from build123d import *

# Parameters (mm, degrees)
F0_R     = 40
F1_DEPTH = 10
F2_SIZE  = 2
F3_R     = 22.145473903
F4_DEPTH = 25
F6_D     = 10
F7_R     = 2
F8_SIZE  = 5


with BuildPart() as f1:
    # F0 (on Top) → F1 (new body)
    with BuildSketch(Plane.XY):
        with Locations((-1.4435499907, 0.3608763218)):
            Circle(F0_R)
    extrude(amount=F1_DEPTH)

    # F2
    f2_edges = [f1.edges().sort_by_distance(p)[0] for p in [
        (-41.44355, 0.360876, 10),
    ]]
    chamfer(f2_edges, length=F2_SIZE)

    # F3 (on face) → F4 (join)
    with BuildSketch(Plane.XY.offset(10)):
        Circle(F3_R)
    extrude(amount=F4_DEPTH)

    # F6 (through all)
    with Locations(Plane.XY.offset(35)):
        with Locations((0, 0)):
            Hole(F6_D / 2)

    # F7
    f7_edges = [f1.edges().sort_by_distance(p)[0] for p in [
        (-41.44355, 0.360876, 0),
        (-22.145474, 0, 35),
        (-5, 0, 0),
    ]]
    fillet(f7_edges, radius=F7_R)

    # F8
    f8_edges = [f1.edges().sort_by_distance(p)[0] for p in [
        (22.145474, 0, 21.5),
        (-22.145474, 0, 33),
        (-22.145474, 0, 10),
    ]]
    chamfer(f8_edges, length=F8_SIZE)


solid = f1.part
Read the model definition and answer for the solid it produces. Units are mm, in the model's axes. A direction names the side the tool comes from. Coordinates: 2 decimals unless noted, no trailing zeros. Write each loop counter-clockwise with the first axis right and the second up, starting at its lowest first coordinate (ties: lowest second). Pieces come first, ordered by that corner, then holes. Notation, with made-up numbers: (86, -1.5) -> (96, -1.5) arc R13 ccw to (96, 12.5) -> close; hole circle Ø7 at (-21, -23). An arc over 180 degrees is marked (long way). Return JSON: item names as keys, results as strings.
(1) Each of these flat-tipped pins is pushed along its axis until it touches: P1, Ø1, axis at y = 13, z = 20.5, coming from the -X side; P2, Ø10, axis at y = 21, z = 28, coming from the +X side; P3, Ø10, axis at x = 24, z = 28.5, coming from the -Y side. Where does it stop, or does it pass through?
Answers below:
{"P1": "x = -18.28", "P2": "x = 15.31", "P3": "y = -11.38"}
(2) Consider line 1 along Y through (x, z) = (0, 15); line 2 along Z through (x, y) = (-23, 15.5); line 3 along Y through (x, z) = (-3.5, 11). Determine where each line is inside the solid, lowest interval first. Write a range as from..to.
Answers below:
{"line 1": "-22.15..-5, 5..22.15", "line 2": "0..10", "line 3": "-25.91..-3.57, 3.57..25.91"}
(3) The part is cut by section B-B on z = 3.5. Give the vertices of the cut face in (x, y).
Answers below:
{"outline": "circle Ø80 at (-1.44, 0.36); hole circle Ø10 at (0, 0)"}
(4) The part is cut by section A-A on z = 19. Give the vertices of the cut face in (x, y), then the cut area to 3 significant figures.
Answers below:
{"outline": "circle Ø44.29 at (0, 0); hole circle Ø10 at (0, 0)", "area": "1,460 mm^2"}
(5) Which of the six approach directions +Z, -Z, +X, -X, +Y, -Y give full straight-line access (tool end or side, diameter ignored) to faces 1 (the flat face through (-27.3, 0.9, 10)), 2 (the cylindrical face through (-10.11, -38.69, 4.96))?
Answers below:
{"face 1": "+Z", "face 2": "+Z, -Z"}
(6) For a pull along X with two mould halves and no side action, classify faces 3 (the cylindrical face through (21.123, 6.652, 23.874)), 4 (the cylindrical face through (1.08, -4.88, 18.27)), 5 (the flat face through (4, -4, 35)) as pulls with the +X half, pulls with the -X half, needs draft (parallel to the pull), parting line crosses it, or undercut.
Answers below:
{"face 3": "parting line crosses it", "face 4": "undercut", "face 5": "needs draft"}
